Autodesk Inventor part; units mm, degrees
ref_plane "YZ Plane" through (0, 0, 0) normal (1, 0, 0) x (0, 1, 0)
ref_plane "XZ Plane" through (0, 0, 0) normal (0, 1, 0) x (-1, 0, 0)
ref_plane "XY Plane" through (0, 0, 0) normal (0, 0, 1) x (1, 0, 0)
sketch "Sketch1" plane through (0, 0, 0) normal (0, 0, 1) x (1, 0, 0)
  circle A0 centre (0, 0) radius 142.621
  circle A1 centre (0, 0) radius 162.56
  circle A2 centre (0, 0) radius 132.461
  dimension "d0" = 285.242
  dimension "d1" = 325.12
  dimension "d2" = 264.922
extrude "Extrusion1" add sketch "Sketch1" against normal blind 6.096 contours A0 | A1
extrude "Extrusion2" add sketch "Sketch1" along normal blind 6.096 contours A1
properties part number "outer piece"
Work out the finished part from the listing and answer in its coordinate system (mm). A direction names the side the tool comes from. Round coordinates to 2 decimals unless told otherwise and drop trailing zeros. Loops run counter-clockwise (first coordinate to the right, second up) from the corner with the lowest first, then second, coordinate; pieces in that order, holes last.
(1) The part is cut by section A-A, the plane y = 0. Give the vertices of the cut face in (x, z).
Computed values:
outline: (-162.56, -6.1) - (-132.46, -6.1) - (-132.46, 0) - (-142.62, 0) - (-142.62, 6.1) - (-162.56, 6.1) - close; (132.46, -6.1) - (162.56, -6.1) - (162.56, 6.1) - (142.62, 6.1) - (142.62, 0) - (132.46, 0) - close
(2) The part is cut by section C-C, the plane z = -2.5. Give the vertices of the cut face in (x, y).
Computed values:
outline: circle Ø325.12 at (0, 0); hole circle Ø264.92 at (0, 0)
(3) Each of these flat-tipped pins is pushed along its axis until it touches: P1, Ø6, axis at x = -91, z = 1, coming from the -Y side; P2, Ø1, axis at y = -103.5, z = -4.5, coming from the +X side; P3, Ø1, axis at x = -119, z = 2, coming from the +Y side. Where does it stop, or does it pass through?
Computed values:
P1: stops at y = -136.68
P2: stops at x = 125.76
P3: stops at y = 111.28
(4) The mould has two halves that part along Y. Classify faces 3 (the cylindrical face through (-21.162, -161.177, -0.085)), 4 (the flat face through (-133, 1, -6.096)), 5 (the cylindrical face through (-105.117, -80.6, -3.005)), 6 (the flat face through (42, -126, 0)): pulls with the +Y half, pulls with the -Y half, needs draft (parallel to the pull), parting line crosses it, or undercut.
Computed values:
face 3: parting line crosses it
face 4: needs draft
face 5: undercut
face 6: undercut
(5) Find the intervals of material crossed by L1, parallel to Y at x = 0, z = 1.75; L2, parallel to Y at x = 0, z = -2.5; L3, parallel to Z at x = 12.5, y = 136, in increasing order.
Computed values:
L1: y = -162.56 to -142.62, 142.62 to 162.56
L2: y = -162.56 to -132.46, 132.46 to 162.56
L3: z = -6.1 to 0
(6) For faces 1 (the flat face through (-1, -144, 6.096)), 2 (the cylindrical face through (-105.12, -96.39, 3.01)), determine the directions among +Z, -Z, +X, -X, +Y, -Y from which every point of the face is accessible in a straight line to the end or side of a thin tool.
Computed values:
face 1: +Z, +X, -X, +Y, -Y
face 2: +Z
